```python
from build123d import *

# Parameters (mm, degrees)
SKETCH1_R                = 76.2
BOSS_EXTRUDE1_DEPTH      = 3.175
BOSS_EXTRUDE2_DEPTH      = 3.175
SKETCH3_R                = 4
BOSS_EXTRUDE3_DEPTH      = 12.954
BOSS_EXTRUDE3_DEPTH_BACK = 6.35
CUT_EXTRUDE1_DEPTH       = 4.175


with BuildPart() as part:
    # Sketch1 → Boss-Extrude1 (new body)
    with BuildSketch(Plane(origin=(0, 0, 0), x_dir=(1, 0, 0), z_dir=(0, 1, 0))):
        Circle(SKETCH1_R)
    extrude(amount=BOSS_EXTRUDE1_DEPTH)

    # Sketch2 → Boss-Extrude2 (add)
    with BuildSketch(Plane(origin=(0, 3.175, 0), x_dir=(1, 0, 0), z_dir=(0, 1, 0))):
        with BuildLine():
            Line((-74.676, 1.524), (74.676, 1.524))
            ThreePointArc((74.676, 1.524), (76.2, 0), (74.676, -1.524))
            Line((74.676, -1.524), (-74.676, -1.524))
            ThreePointArc((-74.676, -1.524), (-76.2, 0), (-74.676, 1.524))
        make_face()
        with BuildLine():
            Line((1.4605, 74.7395), (1.4605, -74.7395))
            ThreePointArc((1.4605, -74.7395), (0, -76.2), (-1.4605, -74.7395))
            Line((-1.4605, -74.7395), (-1.4605, 74.7395))
            ThreePointArc((-1.4605, 74.7395), (0, 76.2), (1.4605, 74.7395))
        make_face()
    extrude(amount=BOSS_EXTRUDE2_DEPTH)

    # Sketch3 → Boss-Extrude3 (add, two sides)
    with BuildSketch(Plane(origin=(0, 6.35, 0), x_dir=(1, 0, 0), z_dir=(0, 1, 0))) as boss_extrude3_sk:
        Circle(SKETCH3_R)
    extrude(amount=BOSS_EXTRUDE3_DEPTH)
    extrude(boss_extrude3_sk.sketch, amount=-BOSS_EXTRUDE3_DEPTH_BACK)

    # Sketch4 → Cut-Extrude1 (cut, through all)
    with BuildSketch(Plane(origin=(0, 3.175, 0), x_dir=(1, 0, 0), z_dir=(0, 1, 0))):
        with BuildLine():
            Line((-7.8105, 7.874), (-39.5605, 7.874))
            Line((-39.5605, 7.874), (-63.009920838, 7.874))
            Line((-63.009920838, 7.874), (-66.208426571, 7.874))
            ThreePointArc((-66.208426571, 7.874), (-47.123731651, 47.168946779), (-7.8105, 66.215947586))
            Line((-7.8105, 66.215947586), (-7.8105, 63.017823588))
            Line((-7.8105, 63.017823588), (-7.8105, 7.874))
        make_face()
        with BuildLine():
            Line((7.874, 63.009920838), (7.874, 66.208426571))
            ThreePointArc((7.874, 66.208426571), (47.168946779, 47.123731651), (66.215947586, 7.8105))
            Line((66.215947586, 7.8105), (63.017823588, 7.8105))
            Line((63.017823588, 7.8105), (7.874, 7.8105))
            Line((7.874, 7.8105), (7.874, 39.5605))
            Line((7.874, 39.5605), (7.874, 63.009920838))
        make_face()
        with BuildLine():
            Line((63.009920838, -7.874), (66.208426571, -7.874))
            ThreePointArc((66.208426571, -7.874), (47.123731651, -47.168946779), (7.8105, -66.215947586))
            Line((7.8105, -66.215947586), (7.8105, -63.017823588))
            Line((7.8105, -63.017823588), (7.8105, -7.874))
            Line((7.8105, -7.874), (39.5605, -7.874))
            Line((39.5605, -7.874), (63.009920838, -7.874))
        make_face()
        with BuildLine():
            Line((-7.874, -63.009920838), (-7.874, -66.208426571))
            ThreePointArc((-7.874, -66.208426571), (-47.168946779, -47.123731651), (-66.215947586, -7.8105))
            Line((-66.215947586, -7.8105), (-63.017823588, -7.8105))
            Line((-63.017823588, -7.8105), (-7.874, -7.8105))
            Line((-7.874, -7.8105), (-7.874, -39.5605))
            Line((-7.874, -39.5605), (-7.874, -63.009920838))
        make_face()
    extrude(amount=-CUT_EXTRUDE1_DEPTH, mode=Mode.SUBTRACT)


solid = part.part
```
The listing builds one solid part. Answer for the finished solid, in the listing's coordinates (mm). A direction names the side the tool comes from. Round coordinates to 2 decimals unless told otherwise and drop trailing zeros. Loops run counter-clockwise (first coordinate to the right, second up) from the corner with the lowest first, then second, coordinate; pieces in that order, holes last.
Q1. Section A-A, the plane z = 36 is taken. Count the separate pieces of the cut face and the enclosed holes in it, then the cut area to 3 significant figures.
Q2. Given pin 1 Ø3.5 at (x, z) = (24, 0.5) entering from +Y; pin 2 Ø1 at (y, z) = (4.5, -51.5) entering from +X; pin 3 Ø1.6 at (x, y) = (36, 5) entering from +Z; pin 4 Ø12 at (x, z) = (43, 41.5) entering from +Y, each flat-ended and moving along its own axis, determine where each tip first touches the part or whether it passes through.
Q3. For a pull along X with two mould halves and no side action, classify faces 1 (the face through (-56, 3.175, -39)), 2 (the face through (-46.73, 1.61, 47.56)), 3 (the face through (-60.47, 1.565, 46.367)) as released by +X, released by -X, zero draft, split by the parting line, or undercut.
Q4. Which of the six approach directions +Z, -Z, +X, -X, +Y, -Y give full straight-line access (tool end or side, diameter ignored) to faces 4 (the face through (49, 3.175, 46)), 5 (the face through (-47.56, 1.61, -46.73)), 6 (the face through (-56, 3.175, 38))?
Q5. Section C-C, the plane y = 13 is taken. Determine the outline of the cut face in (x, z).
Q6. Find the intervals of material crossed by line 1 (X direction, y = 1.75, z = 26); line 2 (X direction, y = 6, z = -46); line 3 (Z direction, x = -19, y = 1), in increasing order.
Completed:
1. separate pieces: 3
1. enclosed holes: 0
1. area: 129 mm2
2. pin 1: stops at y = 6.35
2. pin 2: stops at x = 1.46
2. pin 3: stops at z = 1.52
2. pin 4: passes through
3. face 1: zero draft
3. face 2: undercut
3. face 3: split by the parting line
4. face 4: +Z, +X, +Y
4. face 5: +Y, -Y
4. face 6: +Z, -X, +Y
5. outline: circle Ø8 at (0, 0)
6. line 1: x = -71.63 to -61.4, -7.87 to 7.81, 61.4 to 71.63
6. line 2: x = -1.46 to 1.46
6. line 3: z = -73.79 to -63.91, -7.87 to 7.81, 63.91 to 73.79
